Geometry: final body of the model. Coordinates: model frame, mm. Face numbers are marked on the shaded views. A direction names the side the tool comes from. Coordinates: 2 decimals unless noted, no trailing zeros. Order: outer loops, then holes, each group sorted by start corner. A loop starts at its lowest first (then second) coordinate and runs counter-clockwise, first axis right, second up. Notation, with made-up numbers: (39.5, 67.5) -> (69.5, 67.5) arc R19 ccw to (69.5, 73.5) -> close; hole circle Ø2 at (57, -1). An arc over 180 degrees is marked (long way). Answer in a Markdown table with one row per item. Add a question column.
1) Section query A-A on z = 7.5. Return the cut outline in (x, y).
2) Section query B-B on x = 35. Return the cut outline in (y, z) (3 decimals), then the cut area to 3 significant figures.
3) Section query D-D on x = 7. Return the cut outline in (y, z), then the cut area to 3 significant figures.
4) Pull-direction query (Z, two-part tool) for the marked faces 4, 5 and 6; classes: +Z half, -Z half, draft (parallel to the pull), parting line (faces both ways), or undercut.
5) Ray query, line 1 (X direction, y = 91.5, z = 7.5); line 2 (Z direction, x = 63, y = 94.25); line 3 (Y direction, x = 33.5, z = 10.75). Return the intervals inside material, ascending. Write a range as from..to.
6) Section query C-C on y = 53.5. Return the cut outline in (x, z) (3 decimals), then the cut area to 3 significant figures.
7) Set-up query: the marked faces 1, 2 and 3. Return all of +Z, -Z, +X, -X, +Y, -Y with unobstructed straight access to the full face (end or side cutting, diameter ignored); none if empty.
8) Contact query for flat-ended pins moving along their axis: P1, Ø5, axis at x = 28.5, y = 71, coming from the +Z side; P2, Ø8.5, axis at x = 7, z = 7.5, coming from the +Y side; P3, Ø3.5, axis at x = 27.5, z = 24.5, coming from the +Y side. Output: stop coordinate, or through.
Autodesk Inventor part; units mm, degrees
ref_plane "YZ Plane" through (0, 0, 0) normal (1, 0, 0) x (0, 1, 0)
ref_plane "XZ Plane" through (0, 0, 0) normal (0, 1, 0) x (-1, 0, 0)
ref_plane "XY Plane" through (0, 0, 0) normal (0, 0, 1) x (1, 0, 0)
sketch "Sketch1" plane through (0, 0, 0) normal (0, 0, 1) x (1, 0, 0)
  line L0 (0, 0) -> (70, 0)
  line L1 (70, 0) -> (70, 100)
  line L2 (70, 100) -> (0, 100)
  line L3 (0, 100) -> (0, 0)
  dimension "d0" = 70
  dimension "d1" = 100
extrude "Extrusion1" add sketch "Sketch1" along normal blind 15
sketch "Sketch3" plane through (0, 100, 0) normal (0, 1, 0) x (1, 0, 0)
  line L0 (0, 0) -> (0, -15)
  line L1 (0, -7.5) -> (70, -7.5) construction
  line L2 (70, 0) -> (70, -15)
  circle A0 centre (7, -7.5) radius 4.65
  circle A1 centre (63, -7.5) radius 4.65
  dimension "d7" = 9.3
  dimension "d8" = 9.3
  dimension "d9" = 56
  dimension "d10" = 70
  dimension "d11" = 7
extrude "Extrusion3" cut sketch "Sketch3" against normal blind 15
sketch "Sketch4" plane through (0, 0, 15) normal (0, 0, 1) x (1, 0, 0)
  line L0 (70, 0) -> (70, 100)
  line L1 (0, 0) -> (70, 0)
  line L2 (70, 0) -> (70, 3)
  line L3 (70, 3) -> (0, 3)
  line L4 (0, 3) -> (0, 0)
  dimension "d14" = 3
extrude "Extrusion4" add sketch "Sketch4" along normal blind 15
fillet "Fillet1" radius 4 1 edges at (35, 3, 15)
sketch "Sketch5" plane through (0, 0, 15) normal (0, 0, 1) x (1, 0, 0)
  line L0 (70, 0) -> (70, 100)
  line L1 (0, 0) -> (70, 0)
  line L2 (0, 100) -> (0, 0)
  line L3 (70, 100) -> (0, 100)
  circle A0 centre (35, 53.5) radius 4.625
  line L4 (70, 100) -> (0, 100)
  line L5 (35, 100) -> (35, 0)
  line L6 (0, 0) -> (70, 0)
  line L7 (70, 7) -> (70, 100)
  line L8 (70, 53.5) -> (0, 53.5)
  line L9 (0, 100) -> (0, 7)
  dimension "d18" = 9.25
sketch "Sketch5 outline for Extrusion5" plane through (0, 0, 15) normal (0, 0, 1) x (1, 0, 0)
  circle A0 centre (35, 53.5) radius 4.625
extrude "Extrusion5" cut sketch "Sketch5 outline for Extrusion5" against normal blind 11 draft -2
equation "\"d8\" = d7"
equation "\"d11\" = -0.5 * d9 + 0.5 * d10"
properties part number "antenna_mast_mount"
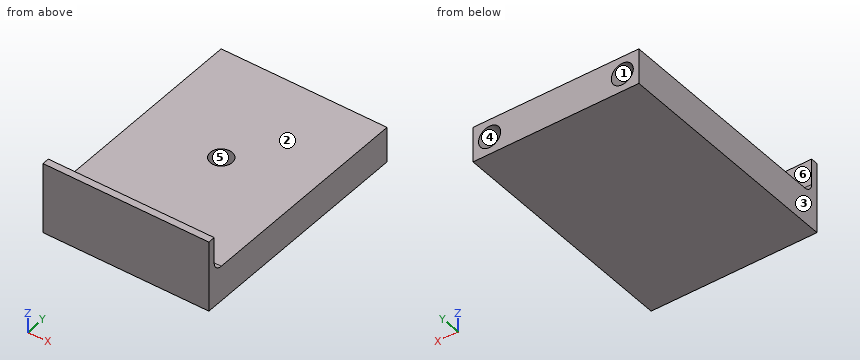
Result:
| question | item | result |
|---|---|---|
| 1 | outline | (0, 0) -> (70, 0) -> (70, 100) -> (67.65, 100) -> (67.65, 85) -> (58.35, 85) -> (58.35, 100) -> (11.65, 100) -> (11.65, 85) -> (2.35, 85) -> (2.35, 100) -> (0, 100) -> close; hole circle Ø8.73 at (35, 53.5) |
| 2 | outline | (0, 0) -> (100, 0) -> (100, 15) -> (58.125, 15) -> (57.741, 4) -> (49.259, 4) -> (48.875, 15) -> (7, 15) arc R4 cw to (3, 19) -> (3, 30) -> (0, 30) -> close |
| 2 | area | 1,450 mm2 |
| 3 | outline | (0, 0) -> (100, 0) -> (100, 2.85) -> (85, 2.85) -> (85, 12.15) -> (100, 12.15) -> (100, 15) -> (7, 15) arc R4 cw to (3, 19) -> (3, 30) -> (0, 30) -> close |
| 3 | area | 1,410 mm2 |
| 4 | face 4 | undercut |
| 4 | face 5 | +Z half |
| 4 | face 6 | draft |
| 5 | line 1 | 0..2.35, 11.65..58.35, 67.65..70 |
| 5 | line 2 | 0..2.85, 12.15..15 |
| 5 | line 3 | 0..49.28, 57.72..100 |
| 6 | outline | (0, 0) -> (70, 0) -> (70, 15) -> (39.625, 15) -> (39.241, 4) -> (30.759, 4) -> (30.375, 15) -> (0, 15) -> close |
| 6 | area | 952 mm2 |
| 7 | face 1 | +Y |
| 7 | face 2 | +Z, +X, -X, +Y |
| 7 | face 3 | +Z, -Z, -X, +Y, -Y |
| 8 | P1 | z = 15 |
| 8 | P2 | y = 85 |
| 8 | P3 | y = 3 |
